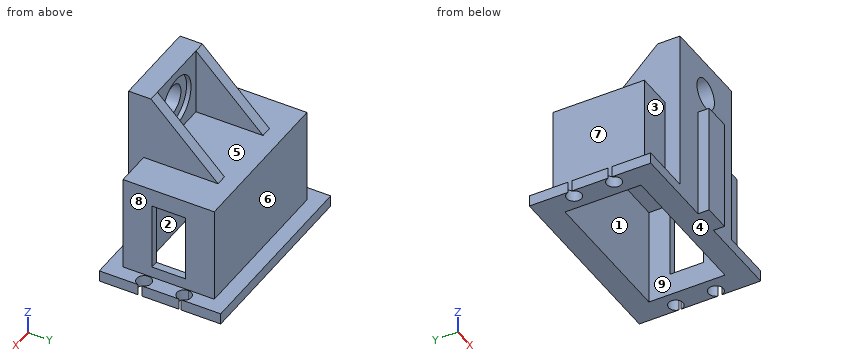
```python
from build123d import *

# Parameters (mm, degrees)
SKETCH1_W           = 54.356
SKETCH1_H           = 34.4678
SKETCH1_W_2         = 40.2082
SKETCH1_H_2         = 20.32
BOSS_EXTRUDE1_DEPTH = 27.94
SKETCH2_W           = 54.356
SKETCH2_H           = 34.4678
SKETCH2_W_2         = 45.7962
SKETCH2_H_2         = 25.908
CUT_EXTRUDE1_DEPTH  = 24.765
SKETCH3_R           = 2.04968225
SKETCH3_R_2         = 2.0955
CUT_EXTRUDE2_DEPTH  = 43.618007851
SKETCH4_W           = 19.05
SKETCH4_H           = 9.525
CUT_EXTRUDE3_DEPTH  = 12.7
SKETCH5_W           = 45.7962
SKETCH5_H           = 25.908
BOSS_EXTRUDE2_DEPTH = 2.54
SKETCH6_W           = 25.4
SKETCH6_H           = 4.2799
BOSS_EXTRUDE3_DEPTH = 27.305
SKETCH7_W           = 25.4
SKETCH7_H           = 6.35
BOSS_EXTRUDE4_DEPTH = 19.05
SKETCH8_R           = 4.318
CUT_EXTRUDE4_DEPTH  = 19.05
SKETCH9_R           = 7.112
CUT_EXTRUDE5_DEPTH  = 1.27
SKETCH10_W          = 3.175
SKETCH10_H          = 19.05
BOSS_EXTRUDE5_DEPTH = 19.05
CHAMFER1_SIZE       = 19.05
SKETCH12_W          = 7.62
SKETCH12_H          = 31.75
BOSS_EXTRUDE6_DEPTH = 3.175
SKETCH13_W          = 41.4782
SKETCH13_H          = 21.59
CUT_EXTRUDE7_DEPTH  = 27.94


with BuildPart() as part:
    # Sketch1 → Boss-Extrude1 (new body)
    with BuildSketch(Plane.XY):
        Rectangle(SKETCH1_W, SKETCH1_H)
        Rectangle(SKETCH1_W_2, SKETCH1_H_2, mode=Mode.SUBTRACT)
    extrude(amount=-BOSS_EXTRUDE1_DEPTH)

    # Sketch2 → Cut-Extrude1 (cut)
    with BuildSketch(Plane.XY):
        Rectangle(SKETCH2_W, SKETCH2_H)
        Rectangle(SKETCH2_W_2, SKETCH2_H_2, mode=Mode.SUBTRACT)
    extrude(amount=-CUT_EXTRUDE1_DEPTH, mode=Mode.SUBTRACT)

    # Sketch3 → Cut-Extrude2 (cut, through all)
    with BuildSketch(Plane(origin=(0, 0, -27.94), x_dir=(-1, 0, 0), z_dir=(0, 0, -1))):
        with Locations((-25.146, 5.6769)):
            Circle(SKETCH3_R)
        with Locations((-25.146, -5.6769)):
            Circle(SKETCH3_R_2)
        with Locations((25.146, -5.6769)):
            Circle(SKETCH3_R_2)
        with Locations((25.146, 5.6769)):
            Circle(SKETCH3_R_2)
    extrude(amount=-CUT_EXTRUDE2_DEPTH, mode=Mode.SUBTRACT)

    # Sketch4 → Cut-Extrude3 (cut)
    with BuildSketch(Plane(origin=(22.8981, 0, 0), x_dir=(0, 0, -1), z_dir=(1, 0, 0))):
        with Locations((12.065, 0)):
            Rectangle(SKETCH4_W, SKETCH4_H)
    extrude(amount=-CUT_EXTRUDE3_DEPTH, mode=Mode.SUBTRACT)

    # Sketch5 → Boss-Extrude2 (add)
    with BuildSketch(Plane.XY):
        Rectangle(SKETCH5_W, SKETCH5_H)
    extrude(amount=BOSS_EXTRUDE2_DEPTH)

    # Sketch6 → Boss-Extrude3 (add)
    with BuildSketch(Plane.XY.offset(2.54)):
        with Locations((0, -15.09395)):
            Rectangle(SKETCH6_W, SKETCH6_H)
    extrude(amount=-BOSS_EXTRUDE3_DEPTH)

    # Sketch7 → Boss-Extrude4 (add)
    with BuildSketch(Plane.XY.offset(2.54)):
        with Locations((0, -14.0589)):
            Rectangle(SKETCH7_W, SKETCH7_H)
    extrude(amount=BOSS_EXTRUDE4_DEPTH)

    # Sketch8 → Cut-Extrude4 (cut)
    with BuildSketch(Plane(origin=(0, -10.8839, 0), x_dir=(1, 0, 0), z_dir=(0, 1, 0))):
        with Locations(Location((0, -12.065, 0), (0, 0, 270))):
            Circle(SKETCH8_R)
    extrude(amount=-CUT_EXTRUDE4_DEPTH, mode=Mode.SUBTRACT)

    # Sketch9 → Cut-Extrude5 (cut)
    with BuildSketch(Plane(origin=(0, -10.8839, 0), x_dir=(1, 0, 0), z_dir=(0, 1, 0))):
        with Locations(Location((0, -12.065, 0), (0, 0, 270))):
            Circle(SKETCH9_R)
    extrude(amount=-CUT_EXTRUDE5_DEPTH, mode=Mode.SUBTRACT)

    # Sketch10 → Boss-Extrude5 (add)
    with BuildSketch(Plane(origin=(0, -10.8839, 0), x_dir=(1, 0, 0), z_dir=(0, 1, 0))):
        with Locations((11.1125, -12.065)):
            Rectangle(SKETCH10_W, SKETCH10_H)
        with Locations((-11.1125, -12.065)):
            Rectangle(SKETCH10_W, SKETCH10_H)
    extrude(amount=BOSS_EXTRUDE5_DEPTH)

    # Chamfer1
    chamfer1_edges = [part.edges().sort_by_distance(p)[0] for p in [
        (-11.1125, 8.1661, 21.59),
        (11.1125, 8.1661, 21.59),
    ]]
    chamfer(chamfer1_edges, length=CHAMFER1_SIZE - 0.0001)  # a hair under: the kernel refuses the full size

    # Sketch12 → Boss-Extrude6 (add)
    with BuildSketch(Plane.XZ.offset(17.2339)):
        with Locations((0, -12.065)):
            Rectangle(SKETCH12_W, SKETCH12_H)
    extrude(amount=BOSS_EXTRUDE6_DEPTH)

    # Sketch13 → Cut-Extrude7 (cut)
    with BuildSketch(Plane(origin=(0, 0, -27.94), x_dir=(-1, 0, 0), z_dir=(0, 0, -1))):
        Rectangle(SKETCH13_W, SKETCH13_H)
    extrude(amount=-CUT_EXTRUDE7_DEPTH, mode=Mode.SUBTRACT)


solid = part.part
```
Input: part model. Units: mm. Frame: model coordinates. Face numbers are marked on the shaded views. A direction names the side the tool comes from. Coordinates: 2 decimals unless noted, no trailing zeros. Loops run counter-clockwise (first coordinate to the right, second up) from the corner with the lowest first, then second, coordinate; pieces in that order, holes last.
Q1. Contact query for flat-ended pins moving along their axis: pin 1 (6 mm diameter, centred on x = -17.5, y = -11.5, fed in from +Z); pin 2 (11.5 mm diameter, centred on x = 0, z = 14, fed in from +Y); pin 3 (1.5 mm diameter, centred on y = -2, z = -14, fed in from +X). Output: stop coordinate, or through.
Results are:
pin 1: stops at z = 2.54
pin 2: stops at y = -10.88
pin 3: stops at x = -20.74
Q2. Section D-D, the plane z = 9.5. Return the cut outline in (x, y) (3 decimals), and give its area (3 significant figures).
Results are:
outline: (-12.7, -17.234) - (-3.474, -17.234) - (-3.474, -12.154) - (-6.633, -12.154) - (-6.633, -10.884) - (-9.525, -10.884) - (-9.525, 1.206) - (-12.7, 1.206) - close; (3.474, -17.234) - (12.7, -17.234) - (12.7, 1.206) - (9.525, 1.206) - (9.525, -10.884) - (6.633, -10.884) - (6.633, -12.154) - (3.474, -12.154) - close
area: 186 mm2
Q3. Section C-C, the plane x = -8.5. Return the cut outline in (y, z) (3 decimals), and give its area (3 significant figures).
Results are:
outline: (-17.234, -27.94) - (-10.795, -27.94) - (-10.795, 0) - (10.795, 0) - (10.795, -27.94) - (17.234, -27.94) - (17.234, -24.765) - (12.954, -24.765) - (12.954, 2.54) - (-10.884, 2.54) - (-10.884, 21.59) - (-17.234, 21.59) - close
area: 451 mm2
Q4. Mould query, pull axis Y, two halves, no side actions, for the marked faces 1, 2, 3 and 4. Classes: +Y half, -Y half, draft (parallel to the pull), parting line (faces both ways), or undercut.
Results are:
face 1: undercut
face 2: undercut
face 3: -Y half
face 4: draft
Q5. Section B-B, the plane y = 10. Return the cut outline in (x, z) (3 decimals), and give its area (3 significant figures).
Results are:
outline: (-27.178, -27.94) - (-20.739, -27.94) - (-20.739, 0) - (20.739, 0) - (20.739, -27.94) - (27.178, -27.94) - (27.178, -24.765) - (22.898, -24.765) - (22.898, 2.54) - (-22.898, 2.54) - (-22.898, -24.765) - (-27.178, -24.765) - close
area: 264 mm2
Q6. Set-up query: the marked faces 5, 6, 7, 8 and 9. Return all of +Z, -Z, +X, -X, +Y, -Y with unobstructed straight access to the full face (end or side cutting, diameter ignored); none if empty.
Results are:
face 5: +Z, +Y
face 6: +Z, +X, -X, +Y
face 7: +Z, -X, +Y, -Y
face 8: +Z, +X, +Y, -Y
face 9: -Z
Q7. Section A-A, the plane x = 0. Return the cut outline in (y, z) (3 decimals).
Results are:
outline: (-20.409, -27.94) - (-10.795, -27.94) - (-10.795, 0) - (10.795, 0) - (10.795, -27.94) - (17.234, -27.94) - (17.234, -24.765) - (12.954, -24.765) - (12.954, 2.54) - (-10.884, 2.54) - (-10.884, 4.953) - (-12.154, 4.953) - (-12.154, 7.747) - (-17.234, 7.747) - (-17.234, 3.81) - (-20.409, 3.81) - close; (-17.234, 16.383) - (-12.154, 16.383) - (-12.154, 19.177) - (-10.884, 19.177) - (-10.884, 21.59) - (-17.234, 21.59) - close
Q8. Line query: line 1 along Y through (x, z) = (22.5, -12.5); line 2 along X through (y, z) = (6.5, -16.5); line 3 along Y through (x, z) = (-4, -2) (3 decimals). Output: solid intervals per line, ascending.
Results are:
line 1: y = -12.95 to -4.76, 4.76 to 12.95
line 2: x = -22.9 to -20.74, 20.74 to 22.9
line 3: y = -17.234 to -10.795, 10.795 to 12.954
